CAD build for the part. Positions are in the model's coordinates, mm. A direction names the side the tool comes from. Coordinates: 2 decimals unless noted, no trailing zeros. Order: outer loops, then holes, each group sorted by start corner. A loop starts at its lowest first (then second) coordinate and runs counter-clockwise, first axis right, second up. Notation, with made-up numbers: (50.25, -27.75) - (109.25, -27.75) arc R31 ccw to (109.25, 5.25) - close; hole circle Ø4 at (-25.75, -15). An arc over 180 degrees is marked (long way). Return JSON: item names as keys, results as strings.
from build123d import *

# Parameters (mm, degrees)
BOSS_EXTRUDE1_DEPTH = 3
BOSS_EXTRUDE2_DEPTH = 2.5
SKETCH4_W           = 2
SKETCH4_H           = 2.442088572
FILLET1_R           = 1
FILLET2_R           = 1
CUT_EXTRUDE2_DEPTH  = 5
SKETCH6_W           = 34.8
SKETCH6_H           = 8
BOSS_EXTRUDE3_DEPTH = 3


with BuildPart() as part:
    # Sketch2 → Boss-Extrude1 (new, symmetric)
    with BuildSketch(Plane(origin=(0, 0, 0), x_dir=(0, 0, -1), z_dir=(1, 0, 0))):
        Polygon((0, 0), (40, 0), (40, 12.4), (45, 12.4), (45, -5), (0, -5), align=None)
    extrude(amount=BOSS_EXTRUDE1_DEPTH, both=True)

    # Sketch3 → Boss-Extrude2 (add, symmetric)
    with BuildSketch(Plane.XY):
        with BuildLine():
            Line((-3, 2.442088572), (-3, -5))
            Line((-3, -5), (3, -5))
            Line((3, -5), (3, 2.442088572))
            ThreePointArc((3, 2.442088572), (0, 2), (-3, 2.442088572))
        make_face()
    extrude(amount=BOSS_EXTRUDE2_DEPTH, both=True)

    # Sketch4 → Cut-Revolve1 (revolve, cut)
    with BuildSketch(Plane(origin=(0, 0, 0), x_dir=(0, 0, -1), z_dir=(1, 0, 0))):
        with Locations((0, 1.221044286)):
            Rectangle(SKETCH4_W, SKETCH4_H)
    revolve(axis=Axis((0, 12.4, 0), (0, 0, -1)), mode=Mode.SUBTRACT)

    # Fillet1
    fillet1_edges = [part.edges().sort_by_distance(p)[0] for p in [
        (-3, 2.442088572, 1.75),
        (0, 0, -2.5),
        (3, 2.442088572, 1.75),
        (-3, 2.442088572, -1.75),
        (3, 2.442088572, -1.75),
        (-3, 0.368375006, 0),
        (3, 0.368375006, 0),
    ]]
    fillet(fillet1_edges, radius=FILLET1_R)

    # Fillet2
    # the kernel refuses this fillet: 1 mm, written as the material it adds along each edge
    with BuildSketch(Plane(origin=(0, 12.4, -1), x_dir=(-0.14925373134328332, -0.9887989298538439, 0), z_dir=(-0.9887989298538439, 0.14925373134328332, 0))) as fillet2_piece_1:
        with BuildLine():
            CenterArc((12.4 - FILLET2_R, FILLET2_R), FILLET2_R, 270, 90)
            Line((12.4 - FILLET2_R, 0), (12.4, 0))
            Line((12.4, 0), (12.4, FILLET2_R))
        make_face()
    revolve(axis=Axis((0, 12.4, -1), (0, 0, 1)), revolution_arc=17.167363371)
    with BuildSketch(Plane(origin=(0, 12.4, 1), x_dir=(-0.14925373134328332, -0.9887989298538439, 0), z_dir=(-0.9887989298538439, 0.14925373134328332, 0))) as fillet2_piece_2:
        with BuildLine():
            CenterArc((12.4 - FILLET2_R, -FILLET2_R), FILLET2_R, 0, 90)
            Line((12.4 - FILLET2_R, 0), (12.4, 0))
            Line((12.4, 0), (12.4, -FILLET2_R))
        make_face()
    revolve(axis=Axis((0, 12.4, 1), (0, 0, 1)), revolution_arc=17.167363371)
    with BuildSketch(Plane(origin=(2, -0.84990566, -1), x_dir=(-0.8018642143213413, -0.5975063027205807, 0), z_dir=(-0.5975063027205807, 0.8018642143213413, 0))) as fillet2_piece_3_section:
        with BuildLine():
            CenterArc((1 + FILLET2_R, FILLET2_R), FILLET2_R, 180, 90)
            Line((1, FILLET2_R), (1, 0))
            Line((1, 0), (1 + FILLET2_R, 0))
        make_face()
    fillet2_piece_3 = revolve(axis=Axis((2, -0.84990566, -1), (0, 0, 1)), revolution_arc=241.892173959, mode=Mode.PRIVATE)
    fillet2_piece_3 = split(fillet2_piece_3, bisect_by=Plane(origin=(3, -0.02635607, -0.708719326), z_dir=(-1, 0, 0)), keep=Keep.TOP, mode=Mode.PRIVATE)
    add(fillet2_piece_3)
    with BuildSketch(Plane(origin=(2, -0.84990566, 1), x_dir=(-0.8018642143213406, -0.5975063027205816, 0), z_dir=(-0.5975063027205816, 0.8018642143213406, 0))) as fillet2_piece_4_section:
        with BuildLine():
            CenterArc((1 + FILLET2_R, -FILLET2_R), FILLET2_R, 90, 90)
            Line((1 + FILLET2_R, 0), (1, 0))
            Line((1, 0), (1, -FILLET2_R))
        make_face()
    fillet2_piece_4 = revolve(axis=Axis((2, -0.84990566, 1), (0, 0, 1)), revolution_arc=241.892173959, mode=Mode.PRIVATE)
    fillet2_piece_4 = split(fillet2_piece_4, bisect_by=Plane(origin=(3, -0.026356063, 0.70871933), z_dir=(-1, 0, 0)), keep=Keep.TOP, mode=Mode.PRIVATE)
    add(fillet2_piece_4)
    with BuildSketch(Plane(origin=(-2, -0.84990566, -1), x_dir=(0.8018642143213416, -0.5975063027205804, 0), z_dir=(0.5975063027205804, 0.8018642143213416, 0))) as fillet2_piece_5_section:
        with BuildLine():
            CenterArc((1 + FILLET2_R, -FILLET2_R), FILLET2_R, 90, 90)
            Line((1 + FILLET2_R, 0), (1, 0))
            Line((1, 0), (1, -FILLET2_R))
        make_face()
    fillet2_piece_5 = revolve(axis=Axis((-2, -0.84990566, -1), (0, 0, -1)), revolution_arc=241.892173959, mode=Mode.PRIVATE)
    fillet2_piece_5 = split(fillet2_piece_5, bisect_by=Plane(origin=(-3, -0.026356035, -0.70871925), z_dir=(1, 0, 0)), keep=Keep.TOP, mode=Mode.PRIVATE)
    add(fillet2_piece_5)
    with BuildSketch(Plane(origin=(-2, -0.84990566, 1), x_dir=(0.8018642143213416, -0.5975063027205804, 0), z_dir=(0.5975063027205804, 0.8018642143213416, 0))) as fillet2_piece_6_section:
        with BuildLine():
            CenterArc((1 + FILLET2_R, FILLET2_R), FILLET2_R, 180, 90)
            Line((1 + FILLET2_R, 0), (1, 0))
            Line((1, 0), (1, FILLET2_R))
        make_face()
    fillet2_piece_6 = revolve(axis=Axis((-2, -0.84990566, 1), (0, 0, -1)), revolution_arc=241.892173959, mode=Mode.PRIVATE)
    fillet2_piece_6 = split(fillet2_piece_6, bisect_by=Plane(origin=(-3, -0.026356028, 0.708719255), z_dir=(1, 0, 0)), keep=Keep.TOP, mode=Mode.PRIVATE)
    add(fillet2_piece_6)

    # Sketch5 → Cut-Extrude2 (cut)
    with BuildSketch(Plane.XY.offset(-40)):
        Polygon((3, 6.364466094), (0.5, 12.4), (3, 12.4), align=None)
        Polygon((-0.5, 12.4), (-3, 6.364466094), (-3, 12.4), align=None)
    extrude(amount=-CUT_EXTRUDE2_DEPTH, mode=Mode.SUBTRACT)

    # Sketch6 → Boss-Extrude3 (add, symmetric)
    with BuildSketch(Plane(origin=(0, 0, 0), x_dir=(0, 0, -1), z_dir=(1, 0, 0))):
        with Locations((27.6, -9)):
            Rectangle(SKETCH6_W, SKETCH6_H)
    extrude(amount=BOSS_EXTRUDE3_DEPTH, both=True)


solid = part.part
Item 1: Band-saw the part on C-C, the plane z = -8. List the corners of the cut face in (x, y), then the cut area to 3 significant figures.
Findings below:
{"outline": "(-3, -5) - (3, -5) - (3, 0) - (-3, 0) - close", "area": "30.0 mm²"}
Item 2: Wall check: L1, parallel to Y at x = 1, z = -20; L2, parallel to Z at x = 1.5, y = 3; L3, parallel to Y at x = -0.75, z = -9.5. Give the ranges that are in metal, low to high. Write a range as [from, to].
Findings below:
{"L1": "y = [-13, 0]", "L2": "z = [-45, -40]", "L3": "y = [-5, 0]"}
Item 3: Band-saw the part on B-B, the plane y = -7.75. List the corners of the cut face in (x, z), then the cut area to 3 significant figures.
Findings below:
{"outline": "(-3, -45) - (3, -45) - (3, -10.2) - (-3, -10.2) - close", "area": "209 mm²"}
Item 4: Mould opens along Z. For faces 1 (the flat face through (0, 1.5, 1)), 2 (the flat face through (0, 0, -21)), 3 (the flat face through (0, 0, -45)), 4 (the flat face through (0, -13, -27)) say: released by +Z, released by -Z, zero draft, split by the parting line, or undercut.
Findings below:
{"face 1": "undercut", "face 2": "undercut", "face 3": "released by -Z", "face 4": "zero draft"}
Item 5: Which spindle directions (+Z, -Z, +X, -X, +Y, -Y) get a long thin tool onto all of the face, cutting with end or side? Do faces 5 (the flat face through (0, 1.5, -1)), 6 (the cylindrical face through (0, 2, 2)), 7 (the flat face through (1.767, 9.34, -42.465)), 8 (the flat face through (3, -5, -26)), 9 (the flat face through (0, -5, -4)). Say none if no direction does.
Findings below:
{"face 5": "+X, -X, +Y", "face 6": "+Z, +Y", "face 7": "+Z, -Z, +X, +Y", "face 8": "+Z, -Z, +X, +Y, -Y", "face 9": "+Z, +X, -X, -Y"}
Item 6: Drop flat-ended pins along their axis: P1, Ø1.8, axis at x = -1, y = 5.5, coming from the +Z side; P2, Ø1.8, axis at x = 1, z = -3, coming from the -Y side; P3, Ø5, axis at y = 2, z = -11.5, coming from the -X side. Give the stop position or say it passes through.
Findings below:
{"P1": "stops at z = -40", "P2": "stops at y = -5", "P3": "stops at x = -3"}
Item 7: Band-saw the part on A-A, the plane z = -40.5. List the corners of the cut face in (x, y), then the cut area to 3 significant figures.
Findings below:
{"outline": "(-3, -13) - (3, -13) - (3, 6.36) - (0.5, 12.4) - (-0.5, 12.4) - (-3, 6.36) - close", "area": "137 mm²"}
